Read the model definition and answer for the solid it produces. Units are mm, in the model's axes. Round coordinates to 2 decimals unless told otherwise and drop trailing zeros. Loops run counter-clockwise (first coordinate to the right, second up) from the corner with the lowest first, then second, coordinate; pieces in that order, holes last. Notation, with made-up numbers: M -18,10.25 L 5,10.25 A18 ccw 5,24.25 Z; hole C 74,-38 d5. An arc over 180 degrees is marked long. Answer as CSV lines item,"result".
```python
from build123d import *

# Parameters (mm, degrees)
BOSS_EXTRUDE1_DEPTH = 135
SKETCH2_R           = 1.2
CUT_EXTRUDE1_DEPTH  = 136.273796428


with BuildPart() as part:
    # Sketch1 → Boss-Extrude1 (new body)
    with BuildSketch(Plane.XY):
        Polygon((0, 4), (0, 5), (7, 5), (7, 4), (6.5, 4), (6.5, 3.5), (7, 3.5), (7, 0), (0, 0), (0, 3.5), (0.5, 3.5), (0.5, 4), align=None)
    extrude(amount=BOSS_EXTRUDE1_DEPTH)

    # Sketch2 → Cut-Extrude1 (cut, through all)
    with BuildSketch(Plane(origin=(0, 5, 0), x_dir=(1, 0, 0), z_dir=(0, 1, 0))):
        with Locations(Location((3.5, -130, 0), (0, 0, 270))):
            Circle(SKETCH2_R)
        with Locations(Location((3.5, -115, 0), (0, 0, 270))):
            Circle(SKETCH2_R)
        with Locations(Location((3.5, -100, 0), (0, 0, 270))):
            Circle(SKETCH2_R)
        with Locations(Location((3.5, -85, 0), (0, 0, 270))):
            Circle(SKETCH2_R)
        with Locations(Location((3.5, -70, 0), (0, 0, 270))):
            Circle(SKETCH2_R)
        with Locations(Location((3.5, -55, 0), (0, 0, 270))):
            Circle(SKETCH2_R)
        with Locations(Location((3.5, -40, 0), (0, 0, 270))):
            Circle(SKETCH2_R)
        with Locations(Location((3.5, -25, 0), (0, 0, 270))):
            Circle(SKETCH2_R)
        with Locations(Location((3.5, -10, 0), (0, 0, 270))):
            Circle(SKETCH2_R)
        with Locations((3.5, 5)):
            Circle(SKETCH2_R)
        with Locations((3.5, 20)):
            Circle(SKETCH2_R)
        with Locations((3.5, 35)):
            Circle(SKETCH2_R)
        with Locations((3.5, 50)):
            Circle(SKETCH2_R)
    extrude(amount=-CUT_EXTRUDE1_DEPTH, mode=Mode.SUBTRACT)


solid = part.part
```
1) Straight lines are drawn through the part: line 1 (X direction, y = 3.45, z = 115); line 2 (Y direction, x = 6.75, z = 11); line 3 (X direction, y = 2.2, z = 55.5). For each, find the intervals that lie inside material, in ascending order.
Evaluation:
line 1,"x = 0 to 2.3, 4.7 to 7"
line 2,"y = 0 to 3.5, 4 to 5"
line 3,"x = 0 to 2.41, 4.59 to 7"
2) Find section A-A, the plane z = 25. Give the vertices of the cut face in (x, y).
Evaluation:
outline,"M 0,0 L 2.3,0 L 2.3,5 L 0,5 L 0,4 L 0.5,4 L 0.5,3.5 L 0,3.5 Z; M 4.7,0 L 7,0 L 7,3.5 L 6.5,3.5 L 6.5,4 L 7,4 L 7,5 L 4.7,5 Z"
3) Determine the mould class of faces 1 (the cylindrical face through (3.04, 2.54, 116.11)), 2 (the flat face through (4, 3, 135)), 3 (the cylindrical face through (3.55, 2.54, 23.8)), 4 (the flat face through (7, 2, 67)) for opening direction Z: released by +Z, released by -Z, zero draft, split by the parting line, or undercut.
Evaluation:
face 1,"undercut"
face 2,"released by +Z"
face 3,"undercut"
face 4,"zero draft"
4) Find section B-B, the plane x = 3.5. Count the separate pieces of the cut face and the enclosed holes in it, then the cut area to 3 significant figures.
Evaluation:
separate pieces,"10"
enclosed holes,"0"
area,"567 mm^2"
